Input: dimensioned drawing with shaded views. Units: mm. Origin: part minimum x, y, z. A direction names the side the tool comes from. Round coordinates to 2 decimals unless told otherwise and drop trailing zeros. Write each loop counter-clockwise with the first axis right and the second up, starting at its lowest first coordinate (ties: lowest second). Pieces come first, ordered by that corner, then holes. Notation, with made-up numbers: (25.25, 56.25) - (32.25, 56.25) arc R29 cw to (32.25, 85.25) - close; hole circle Ø1 at (45.5, 34.25). An arc over 180 degrees is marked (long way). Use one line per item in the form item = value.
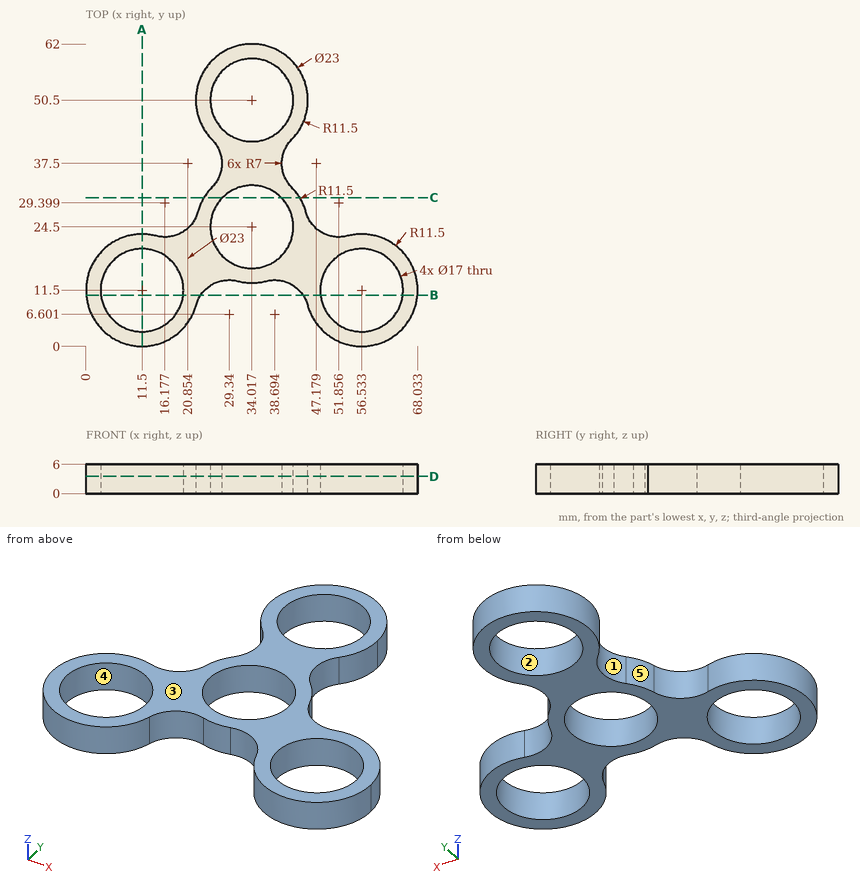
(1) Cut plane A-A on x = 11.5. Output: boundary loops of the cut face in (y, z).
Derived:
outline = (0, 0) - (3, 0) - (3, 6) - (0, 6) - close; (20, 0) - (23, 0) - (23, 6) - (20, 6) - close
(2) First-contact query: pin 1 Ø19.5 at (x, y) = (34.02, 24.5) entering from +Z; pin 2 Ø2 at (y, z) = (23, 1.5) entering from +X (1 decimal); pin 3 Ø1 at (x, z) = (8.5, 3.5) entering from -Y (1 decimal); pin 4 Ø13.5 at (x, y) = (56.53, 11.5) entering from +Z. Flat tips, straight axial feed; report the tip coordinate or a pass-through.
Derived:
pin_1 = 6
pin_2 = 61.2
pin_3 = 0.3
pin_4 = through
(3) Cut plane D-D on z = 3.5. Output: boundary loops of the cut face in (x, y) (1 decimal).
Derived:
outline = (14.4, 22.6) arc R11.5 ccw (long way) to (22.6, 8.5) arc R7 cw to (31.1, 13.4) arc R11.5 ccw to (36.9, 13.4) arc R7 cw to (45.4, 8.5) arc R11.5 ccw (long way) to (53.6, 22.6) arc R7 cw to (45.1, 27.5) arc R11.5 ccw to (42.2, 32.6) arc R7 cw to (42.2, 42.4) arc R11.5 ccw to (45.5, 50.5) arc R11.5 ccw (long way) to (25.8, 42.4) arc R7 cw to (25.8, 32.6) arc R11.5 ccw to (22.9, 27.5) arc R7 cw to start; hole circle Ø17 at (11.5, 11.5); hole circle Ø17 at (34, 24.5); hole circle Ø17 at (34, 50.5); hole circle Ø17 at (56.5, 11.5)
(4) Material intervals for L1, parallel to Y at x = 34, z = 3.95; L2, parallel to Y at x = 57, z = 4.6; L3, parallel to Y at x = 38.5, z = 1.1, sorted ascending.
Derived:
L1 = 13 to 16, 33 to 42, 59 to 62
L2 = 0.01 to 3.01, 19.99 to 22.99
L3 = 13.6 to 17.28, 31.72 to 43.28, 57.72 to 61.09
(5) Draft query along X for the marked faces 1, 2 and 3. Return one class per face: released by +X, released by -X, zero draft, split by the parting line, or undercut.
Derived:
face_1 = released by -X
face_2 = undercut
face_3 = zero draft
(6) Cut plane C-C on y = 30.5. Output: boundary loops of the cut face in (x, z) (1 decimal).
Derived:
outline = (24.2, 0) - (28, 0) - (28, 6) - (24.2, 6) - close; (40, 0) - (43.8, 0) - (43.8, 6) - (40, 6) - close
(7) Access query for the marked faces 4 and 5. Directions: +Z, -Z, +X, -X, +Y, -Y. A direction counts if a zero-diameter tool reaches every point of the face in a straight line with its end or side. Return the directions, or none.
Derived:
face_4 = +Z, -Z
face_5 = +Z, -Z, -X
(8) Cut plane B-B on y = 10.5. Output: boundary loops of the cut face in (x, z) (1 decimal).
Derived:
outline = (0, 0) - (3.1, 0) - (3.1, 6) - (0, 6) - close; (19.9, 0) - (23.5, 0) - (23.5, 6) - (19.9, 6) - close; (44.5, 0) - (48.1, 0) - (48.1, 6) - (44.5, 6) - close; (65, 0) - (68, 0) - (68, 6) - (65, 6) - close
